Here's the drawing with two shaded views (mm, measured from the low corner). I have some questions. A direction names the side the tool comes from. Give positions to 0.01 mm unless a question says otherwise; leave off trailing zeros. Loops run counter-clockwise (first coordinate to the right, second up) from the corner with the lowest first, then second, coordinate; pieces in that order, holes last. Notation, with made-up numbers: M 6,66.5 L 58,66.5 A24 cw 58,76.5 Z; hole C 2,72.25 d2. An arc over 180 degrees is marked long. Write item = value, one per line. Start each with the question number.
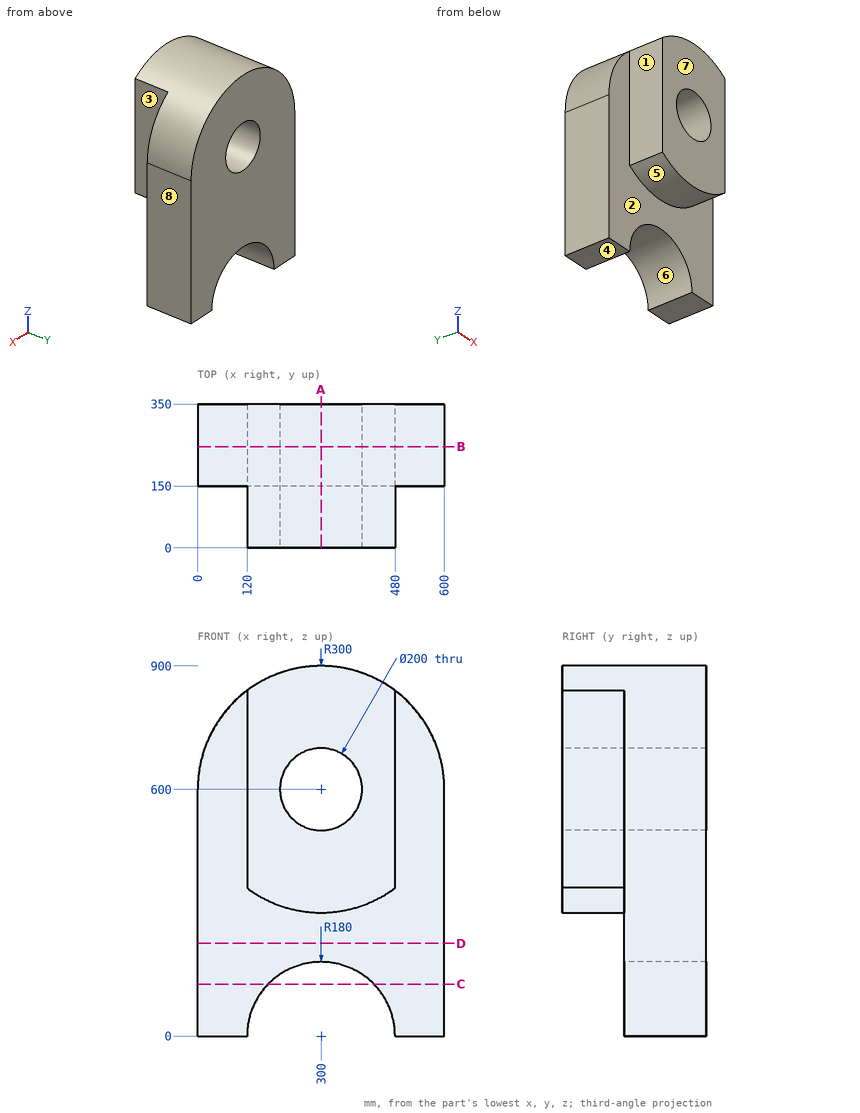
Q1. If we section it at C-C, the plane z = 126: List the corners of the cut face in (x, y) for me, then the cut area to 3 significant figures.
Q2. If I drill on line 1 along Z through (x, y) = (300, 265); line 2 along Z through (x, y) = (294.5, 228); line 3 along Y through (x, z) = (118, 583.5), over which ranges is the centre line in solid material (lowest first)?
Q3. If we section it at D-D, the plane z = 225.5: List the corners of the cut face in (x, y) for me.
Q4. Will these pins go through, and if not, where does the flat tip stop? pin 1 (8 mm diameter, centred on x = 375.5, y = 201.5, fed in from -Z); pin 2 (12 mm diameter, centred on x = 315.5, y = 243.5, fed in from -Z); pin 3 (4 mm diameter, centred on y = 90.5, z = 798.5, fed in from +X); pin 4 (3 mm diameter, centred on x = 282.5, z = 745, fed in from -Y).
Q5. If we section it at B-B, the plane y = 246.5: List the corners of the cut face in (x, z) for me, then the cut area to 3 significant figures.
Q6. We'd pull the mould along X, two halves only. Please class the marked faces 5, 6, 7 and 8: pulls with the +X half, pulls with the -X half, needs draft (parallel to the pull), parting line crosses it, or undercut.
Q7. On a 3-axis mill with a long thin cutter (end or side, diameter ignored), from which of +Z, -Z, +X, -X, +Y, -Y can I reach the whole of each face in a straight line? I mean the marked faces 1, 2, 3 and 4. Say none if no direction works.
Q8. If we section it at A-A, the plane x = 300: List the corners of the cut face in (y, z) for me.
Resolved:
q1.outline = M 0,150 L 171.45,150 L 171.45,350 L 0,350 Z; M 428.55,150 L 600,150 L 600,350 L 428.55,350 Z
q1.area = 68,600 mm²
q2.line_1 = 180 to 500, 700 to 900
q2.line_2 = 179.92 to 500.15, 699.85 to 899.95
q2.line_3 = 150 to 350
q3.outline = M 0,150 L 600,150 L 600,350 L 0,350 Z
q4.pin_1 = 161.49
q4.pin_2 = 178.71
q4.pin_3 = 480
q4.pin_4 = 0
q5.outline = M 0,0 L 120,0 A180 cw 480,0 L 600,0 L 600,600 A300 ccw 0,600 Z; hole C 300,600 d200
q5.area = 419,000 mm²
q6.face_5 = parting line crosses it
q6.face_6 = undercut
q6.face_7 = needs draft
q6.face_8 = pulls with the +X half
q7.face_1 = +Z, -Z, -X, -Y
q7.face_2 = -Z, -Y
q7.face_3 = +Z, -Z, +X, -Y
q7.face_4 = -Z, +X, -X, +Y, -Y
q8.outline = M 0,300 L 150,300 L 150,180 L 350,180 L 350,500 L 0,500 Z; M 0,700 L 350,700 L 350,900 L 0,900 Z
